Check sheet for the modelled part. Datum: model origin and axes. Units: mm. Face numbers are marked on the shaded views. Give positions to 0.01 mm unless a question says otherwise; leave off trailing zeros. Loops run counter-clockwise (first coordinate to the right, second up) from the corner with the lowest first, then second, coordinate; pieces in that order, holes last.
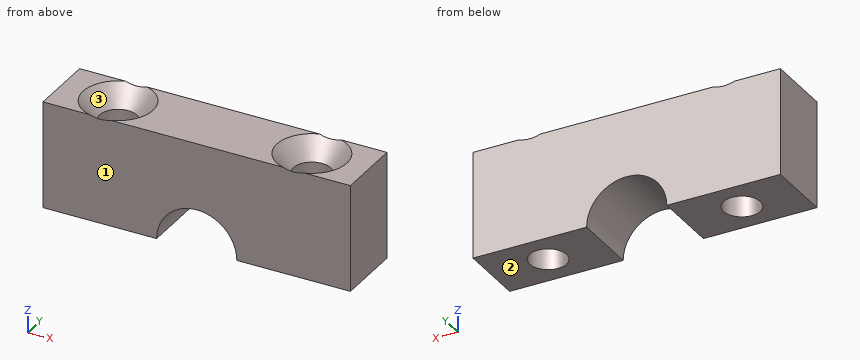
```python
from build123d import *

# Parameters (mm, degrees)
F1_DEPTH       = 25.4
F2_D           = 8.7376
F2_DEPTH       = 29.6333418
F2_CSINK_D     = 16.6624
F2_CSINK_ANGLE = 82
F2_TIP         = 2.6250398724
F4_D           = 19.05


# Not quite as in the source:
# - a feature names something its author has since deleted; it is built from what else it names


with BuildPart() as f1:
    # F0 (on Top) → F1 (new body)
    with BuildSketch(Plane.XY):
        Polygon((36.5125, -7.9375), (36.5125, 7.9375), (0, 7.9375), (-36.5125, 7.9375), (-36.5125, -7.9375), align=None)
    extrude(amount=-F1_DEPTH)

    # F2
    with Locations(Plane.XY):
        with Locations((-23.01875, 0), (23.01875, 0)):
            CounterSinkHole(F2_D / 2, F2_CSINK_D / 2, depth=F2_DEPTH, counter_sink_angle=F2_CSINK_ANGLE)
            with Locations((0, 0, -(F2_DEPTH + F2_TIP / 2))):  # 118° drill point
                Cone(0, F2_D / 2, F2_TIP, mode=Mode.SUBTRACT)

    # F4 (through all)
    with Locations(Plane.XZ.offset(7.9375)):
        with Locations((0, -25.4)):
            Hole(F4_D / 2)


solid = f1.part
```
(1) Material ranges on line 1 (X direction, y = 0, z = -12.5); line 2 (X direction, y = 4.75, z = -2); line 3 (X direction, y = 1.75, z = -21.75), recorded low to high.
(2) Release check for a two-part mould opening along Y. For the marked faces 1, 2 and 3 record: pulls with the +Y half, pulls with the -Y half, needs draft (parallel to the pull), parting line crosses it, or undercut.
(3) Section check B-B on y = 0. Give the number of separate pieces and of enclosed holes in the cut face, plus the area to 3 significant figures.
(4) Section check C-C on z = -18.75. Record the boundary of the cut face in (x, y).
(5) Section check A-A on z = -22.25. Record the boundary of the cut face in (x, y), plus the area to 3 significant figures.
(6) Section check D-D on x = 0. Record the boundary of the cut face in (y, z) (1 decimal).
(7) Gauge pin test, flat end, axial feed: pin 1 Ø1.5 at (x, y) = (-16.5, -0.5) entering from +Z. Record the tip position at first contact, or that the pin passes through.
Computed values:
1. line 1: x = -36.51 to -27.39, -18.65 to 18.65, 27.39 to 36.51
1. line 2: x = -36.51 to -27.59, -18.45 to 18.45, 27.59 to 36.51
1. line 3: x = -36.51 to -27.02, -19.02 to -8.8, 8.8 to 19.02, 27.02 to 36.51
2. face 1: pulls with the -Y half
2. face 2: needs draft
2. face 3: undercut
3. separate pieces: 3
3. enclosed holes: 0
3. area: 1,230 mm2
4. outline: (-36.51, -7.94) - (-6.82, -7.94) - (-6.82, 7.94) - (-36.51, 7.94) - close; (6.82, -7.94) - (36.51, -7.94) - (36.51, 7.94) - (6.82, 7.94) - close; hole circle Ø8.74 at (-23.02, 0); hole circle Ø8.74 at (23.02, 0)
5. outline: (-36.51, -7.94) - (-8.99, -7.94) - (-8.99, 7.94) - (-36.51, 7.94) - close; (8.99, -7.94) - (36.51, -7.94) - (36.51, 7.94) - (8.99, 7.94) - close; hole circle Ø8.74 at (-23.02, 0); hole circle Ø8.74 at (23.02, 0)
5. area: 754 mm2
6. outline: (-7.9, -15.9) - (7.9, -15.9) - (7.9, 0) - (-7.9, 0) - close
7. pin 1: stops at z = -1.2
